Source: CAD feature listing. Evaluate the final solid. Frame: model axes, mm. Face numbers are marked on the shaded views. A direction names the side the tool comes from. Give positions to 0.01 mm unless a question says otherwise; leave off trailing zeros. Write each loop counter-clockwise with the first axis right and the second up, starting at its lowest first coordinate (ties: lowest second). Pieces come first, ordered by that corner, then holes. Notation, with made-up numbers: M -16,39 L 2,39 A24 cw 2,63 Z; hole C -10.75,-13 d3. An arc over 180 degrees is marked long. Return JSON: item names as keys, results as strings.
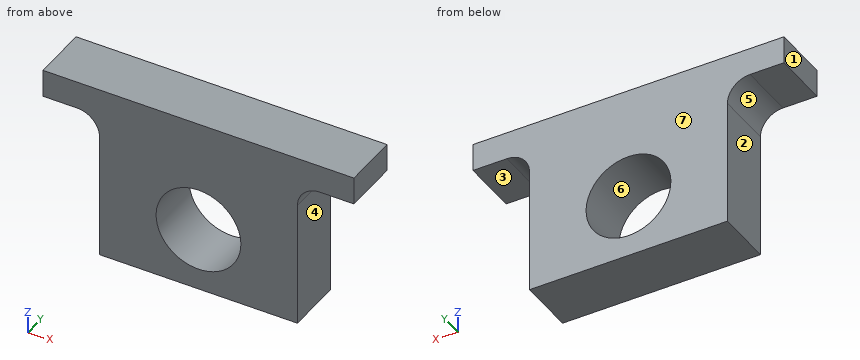
```python
from build123d import *

# Parameters (mm, degrees)
SKETCH1_R           = 9.525
BOSS_EXTRUDE1_DEPTH = 12.7


with BuildPart() as part:
    # Sketch1 → Boss-Extrude1 (new body)
    with BuildSketch(Plane(origin=(0, 0, 0), x_dir=(1, 0, 0), z_dir=(0, 1, 0))):
        with BuildLine():
            Line((22.225, -8.525568981), (22.225, 19.84375))
            Line((22.225, 19.84375), (-22.225, 19.84375))
            Line((-22.225, 19.84375), (-22.225, -8.525568981))
            ThreePointArc((-22.225, -8.525568981), (-23.712897552, -12.117671429), (-27.305, -13.605568981))
            Line((-27.305, -13.605568981), (-34.925, -13.605568981))
            Line((-34.925, -13.605568981), (-34.925, -19.84375))
            Line((-34.925, -19.84375), (34.925, -19.84375))
            Line((34.925, -19.84375), (34.925, -13.605568981))
            Line((34.925, -13.605568981), (27.305, -13.605568981))
            ThreePointArc((27.305, -13.605568981), (23.712897552, -12.117671429), (22.225, -8.525568981))
        make_face()
        with Locations(Location((0, 5.55625, 0), (0, 0, 270))):
            Circle(SKETCH1_R, mode=Mode.SUBTRACT)
    extrude(amount=BOSS_EXTRUDE1_DEPTH)


solid = part.part
```
1) Contact query for flat-ended pins moving along their axis: pin 1 Ø1.5 at (x, z) = (24, 7) entering from +Y; pin 2 Ø6.5 at (y, z) = (9.5, -3.5) entering from +X (3 decimals); pin 3 Ø4 at (x, y) = (32, 5) entering from -Z. Output: stop coordinate, or through.
Numbers:
{"pin 1": "passes through", "pin 2": "stops at x = 22.225", "pin 3": "stops at z = 13.61"}
2) Line query: line 1 (X direction, y = 10, z = -16.5) (3 decimals); line 2 (Z direction, x = 4, y = 10.5); line 3 (X direction, y = 9.75, z = -10.5) (3 decimals). Output: solid intervals per line, ascending. Write a range as [from, to].
Numbers:
{"line 1": "x = [-22.225, 22.225]", "line 2": "z = [-19.84, -14.2], [3.09, 19.84]", "line 3": "x = [-22.225, -8.142], [8.142, 22.225]"}
3) Set-up query: the marked faces 1, 2 and 3. Return all of +Z, -Z, +X, -X, +Y, -Y with unobstructed straight access to the full face (end or side cutting, diameter ignored); none if empty.
Numbers:
{"face 1": "+Z, -Z, -X, +Y, -Y", "face 2": "-Z, -X, +Y, -Y", "face 3": "-Z, +X, +Y, -Y"}
4) Cut plane D-D, the plane z = 7. Return the cut outline in (x, y) (3 decimals).
Numbers:
{"outline": "M -22.225,0 L 22.225,0 L 22.225,12.7 L -22.225,12.7 Z"}
5) Draft query along X for the marked faces 4, 5, 6 and 7. Return one class per face: released by +X, released by -X, zero draft, split by the parting line, or undercut.
Numbers:
{"face 4": "released by +X", "face 5": "released by -X", "face 6": "undercut", "face 7": "zero draft"}
6) Cut plane B-B, the plane y = 8.25. Return the cut outline in (x, z) (3 decimals), then the cut area to 3 significant figures.
Numbers:
{"outline": "M -34.925,13.606 L -27.305,13.606 A5.08 cw -22.225,8.526 L -22.225,-19.844 L 22.225,-19.844 L 22.225,8.526 A5.08 cw 27.305,13.606 L 34.925,13.606 L 34.925,19.844 L -34.925,19.844 Z; hole C 0,-5.556 d19.05", "area": "1,650 mm²"}
7) Cut plane C-C, the plane z = -7.5. Return the cut outline in (x, y) (3 decimals).
Numbers:
{"outline": "M -22.225,0 L -9.325,0 L -9.325,12.7 L -22.225,12.7 Z; M 9.325,0 L 22.225,0 L 22.225,12.7 L 9.325,12.7 Z"}
8) Cut plane A-A, the plane x = 0. Return the cut outline in (y, z).
Numbers:
{"outline": "M 0,-19.84 L 12.7,-19.84 L 12.7,-15.08 L 0,-15.08 Z; M 0,3.97 L 12.7,3.97 L 12.7,19.84 L 0,19.84 Z"}
